Work out the finished part from the listing and answer in its coordinate system (mm). A direction names the side the tool comes from. Give positions to 0.01 mm unless a question says otherwise; leave off trailing zeros. Order: outer loops, then holes, each group sorted by start corner. A loop starts at its lowest first (then second) coordinate and runs counter-clockwise, first axis right, second up. Notation, with made-up numbers: (41, 61.25) - (80, 61.25) arc R30 ccw to (80, 97.25) - close; hole circle Ø5 at (-6, 13.5). An arc over 180 degrees is marked (long way). Put each result on its own line as item: value.
```python
from build123d import *

# Parameters (mm, degrees)
SKETCH_1_R                 = 12
SKETCH_1_R_2               = 2.75
EXTRUDE_1_DEPTH            = 2
SKETCH_2_R                 = 10.5
SKETCH_2_R_2               = 2.75
EXTRUDE_2_DEPTH            = 50
SKETCH_7_W                 = 2.1
SKETCH_7_H                 = 10.5
HOLE_WIZARD_M51_AT_2_COUNT = 2
HOLE_WIZARD_M51_AT_2_PITCH = 10
SKETCH_9_W                 = 2.5
SKETCH_9_H                 = 12
HOLE_WIZARD_M61_AT_2_COUNT = 2
HOLE_WIZARD_M61_AT_2_PITCH = 15


with BuildPart() as part:
    # Эскиз1 → Бобышка-Вытянуть1 (new body)
    with BuildSketch(Plane(origin=(0, 0, 0), x_dir=(1, 0, 0), z_dir=(0, 1, 0))):
        Circle(SKETCH_1_R)
        Circle(SKETCH_1_R_2, mode=Mode.SUBTRACT)
    extrude(amount=EXTRUDE_1_DEPTH)

    # Эскиз2 → Бобышка-Вытянуть2 (add)
    with BuildSketch(Plane(origin=(0, 2, 0), x_dir=(1, 0, 0), z_dir=(0, 1, 0))):
        Circle(SKETCH_2_R)
        Circle(SKETCH_2_R_2, mode=Mode.SUBTRACT)
    extrude(amount=EXTRUDE_2_DEPTH)

    # Эскиз7 → Отверстие обработанное метчиком M51 (revolve, cut)
    with BuildSketch(Plane(origin=(0, 8, 0), x_dir=(0, 1, 0), z_dir=(1, 0, 0))):
        with Locations((1.05, 5.25)):
            Rectangle(SKETCH_7_W, SKETCH_7_H)
    hole_wizard_m51 = revolve(axis=Axis((0, 8, -6.35), (0, 0, 1)), mode=Mode.SUBTRACT)

    # Отверстие обработанное метчиком M51 at 2: Отверстие обработанное метчиком M51 ×2
    with Locations(*[(0, i * HOLE_WIZARD_M51_AT_2_PITCH, 0) for i in range(1, HOLE_WIZARD_M51_AT_2_COUNT)]):
        add(hole_wizard_m51, mode=Mode.SUBTRACT)

    # Эскиз9 → Отверстие обработанное метчиком M61 (revolve, cut)
    with BuildSketch(Plane(origin=(0, 44, 0), x_dir=(0, 1, 0), z_dir=(1, 0, 0))):
        with Locations((1.25, 6)):
            Rectangle(SKETCH_9_W, SKETCH_9_H)
    hole_wizard_m61 = revolve(axis=Axis((0, 44, -6.35), (0, 0, 1)), mode=Mode.SUBTRACT)

    # Отверстие обработанное метчиком M61 at 2: Отверстие обработанное метчиком M61 ×2
    with Locations(*[(0, -i * HOLE_WIZARD_M61_AT_2_PITCH, 0) for i in range(1, HOLE_WIZARD_M61_AT_2_COUNT)]):
        add(hole_wizard_m61, mode=Mode.SUBTRACT)


solid = part.part
```
(1) Section B-B, the plane z = -1.5 is taken. Write down the section's boundary in (x, y).
Geometry check:
outline: (-11.91, 0) - (-2.3, 0) - (-2.3, 52) - (-10.39, 52) - (-10.39, 2) - (-11.91, 2) - close; (2.3, 0) - (11.91, 0) - (11.91, 2) - (10.39, 2) - (10.39, 52) - (2.3, 52) - close
(2) Section D-D, the plane z = 5.5 is taken. Write down the section's boundary in (x, y).
Geometry check:
outline: (-10.67, 0) - (10.67, 0) - (10.67, 2) - (8.94, 2) - (8.94, 52) - (-8.94, 52) - (-8.94, 2) - (-10.67, 2) - close; hole circle Ø5 at (0, 29); hole circle Ø5 at (0, 44); hole circle Ø4.2 at (0, 8); hole circle Ø4.2 at (0, 18)
(3) A tool of negligible diameter and unlimited length cuts with its end or side. For faces 4 (the face through (0, 2, 11)), 5 (the face through (2.22, 45.15, 5.89)), 6 (the face through (-11.99, 0.99, -0.53)), from which of +Z, -Z, +X, -X, +Y, -Y can it reach the whole face along a straight path? Write none if from no direction.
Geometry check:
face 4: +Y
face 5: +Z
face 6: +Y, -Y
(4) Section A-A, the plane x = 0 is taken. Write down the section's boundary in (y, z).
Geometry check:
outline: (0, -12) - (2, -12) - (2, -10.5) - (52, -10.5) - (52, -2.75) - (0, -2.75) - close; (0, 2.75) - (5.9, 2.75) - (5.9, 10.5) - (2, 10.5) - (2, 12) - (0, 12) - close; (10.1, 2.75) - (15.9, 2.75) - (15.9, 10.5) - (10.1, 10.5) - close; (20.1, 2.75) - (26.5, 2.75) - (26.5, 10.5) - (20.1, 10.5) - close; (31.5, 2.75) - (41.5, 2.75) - (41.5, 10.5) - (31.5, 10.5) - close; (46.5, 2.75) - (52, 2.75) - (52, 10.5) - (46.5, 10.5) - close
(5) Section C-C, the plane y = 23 is taken. Write down the section's boundary in (x, z), then the cut area to 3 significant figures.
Geometry check:
outline: circle Ø21 at (0, 0); hole circle Ø5.5 at (0, 0)
area: 323 mm²
(6) Given pin 1 (3.5 mm diameter, centred on x = 0, y = 8, fed in from +Z); pin 2 (4 mm diameter, centred on x = 6, y = 42, fed in from +Z); pin 3 (1 mm diameter, centred on x = 3.5, y = 42, fed in from -Z), each flat-ended and moving along its own axis, determine where each tip first touches the part or whether it passes through.
Geometry check:
pin 1: stops at z = -2.12
pin 2: stops at z = 9.71
pin 3: stops at z = -10.06
(7) Straight lines are drawn through the part: line 1 (Y direction, x = 0, z = 5.75); line 2 (Z direction, x = 0, y = 36.5); line 3 (Y direction, x = -4, z = 10.75). For each, find the intervals that lie inside material, in ascending order.
Geometry check:
line 1: y = 0 to 5.9, 10.1 to 15.9, 20.1 to 26.5, 31.5 to 41.5, 46.5 to 52
line 2: z = -10.5 to -2.75, 2.75 to 10.5
line 3: y = 0 to 2
(8) Determine the mould class of faces 1 (the face through (5.645, 26.65, -8.854)), 2 (the face through (2.2, 52, 2.2)), 3 (the face through (-0.358, 25.636, -2.727)) for opening direction Z: pulls with the +Z half, pulls with the -Z half, needs draft (parallel to the pull), parting line crosses it, or undercut.
Geometry check:
face 1: parting line crosses it
face 2: needs draft
face 3: undercut
